Here's how the part is built. I have some questions about the finished solid (model axes, mm). A direction names the side the tool comes from. Give positions to 0.01 mm unless a question says otherwise; leave off trailing zeros. Loops run counter-clockwise (first coordinate to the right, second up) from the corner with the lowest first, then second, coordinate; pieces in that order, holes last. Notation, with made-up numbers: (-15.75, -6) -> (33.25, -6) arc R22 cw to (33.25, 11) -> close; hole circle Ø2 at (19.25, 58). An arc over 180 degrees is marked (long way). Answer in a Markdown table with one row per item. Add a question column.
Item 1: If we section it at A-A (x = -38.1): Write out the boundary of the cut face in (y, z).
Item 2: For P1, Ø3, axis at x = -21.5, z = 1.5, coming from the +Y side; P2, Ø1.9, axis at x = -72.5, z = 2.5, coming from the -Y side, each with a flat end and sliding along its axis, tell me the tip position at first contact or that it passes through.
Item 3: Which directions (+Z, -Z, +X, -X, +Y, -Y) give clear straight access to the entire face, cutting with the end or side of a thin tool? Please do faces 1 (the face through (-31.75, -3, 3)), 2 (the face through (-64, 39, 6.35)), 3 (the face through (-26, 76.2, 3)).
Item 4: If we section it at B-B (z = 1.5): Give the number of separate pieces and of enclosed holes in the cut face, then the cut area to 3 significant figures.
Item 5: We'd pull the mould along Y, two halves only. Please class faces 4 (the face through (-67, 0, 3)), 5 (the face through (-40.64, 79, 3)), 6 (the face through (-105.863, 70.44, 3.219)): released by +Y, released by -Y, zero draft, split by the parting line, or undercut.
Item 6: If I drill on line 1 (Y direction, x = -108.5, z = 2.5); line 2 (Y direction, x = -25.5, z = 2.75); line 3 (X direction, y = -0.5, z = 1.5), over which ranges is the centre line in solid material (lowest first)?
```python
from build123d import *

# Parameters (mm, degrees)
SKETCH1_W           = 127
SKETCH1_H           = 82.55
SKETCH1_R           = 10.16
SKETCH1_R_2         = 6.985
SKETCH1_W_2         = 25.4
SKETCH1_H_2         = 6.35
SKETCH1_W_3         = 31.75
BOSS_EXTRUDE1_DEPTH = 6.35
SKETCH3_R           = 2.6035
CUT_EXTRUDE1_DEPTH  = 152.604172106
SKETCH4_W           = 27.94
SKETCH4_H           = 6.35
CUT_EXTRUDE2_DEPTH  = 6.35


with BuildPart() as part:
    # Sketch1 → Boss-Extrude1 (new body)
    # profile 1 of 3: a face of its own
    with BuildSketch(Plane.XY):
        with Locations((-63.5, 41.275)):
            Rectangle(SKETCH1_W, SKETCH1_H)
        with Locations((-78.105, 41.275)):
            Circle(SKETCH1_R, mode=Mode.SUBTRACT)
        with Locations((-38.1, 41.275)):
            Circle(SKETCH1_R_2, mode=Mode.SUBTRACT)
    # profile 2 of 3: a face of its own
    with BuildSketch(Plane.XY):
        with Locations((-114.3, -3.175)):
            Rectangle(SKETCH1_W_2, SKETCH1_H_2)
    # profile 3 of 3: a face of its own
    with BuildSketch(Plane.XY):
        with Locations((-15.875, -3.175)):
            Rectangle(SKETCH1_W_3, SKETCH1_H_2)
    extrude(amount=BOSS_EXTRUDE1_DEPTH)

    # Sketch3 → Cut-Extrude1 (cut, through all)
    with BuildSketch(Plane.XY.offset(6.35)):
        with Locations((-108.2675, 71.4375)):
            Circle(SKETCH3_R)
        with Locations((-47.9425, 71.4375)):
            Circle(SKETCH3_R)
        with Locations((-108.2675, 11.1125)):
            Circle(SKETCH3_R)
        with Locations((-47.9425, 11.1125)):
            Circle(SKETCH3_R)
    extrude(amount=-CUT_EXTRUDE1_DEPTH, mode=Mode.SUBTRACT)

    # Sketch4 → Cut-Extrude2 (cut)
    with BuildSketch(Plane(origin=(0, 0, 0), x_dir=(-1, 0, 0), z_dir=(0, 0, -1))):
        with Locations((26.67, 79.375)):
            Rectangle(SKETCH4_W, SKETCH4_H)
    extrude(amount=-CUT_EXTRUDE2_DEPTH, mode=Mode.SUBTRACT)


solid = part.part
```
Recorded:
| question | item | result |
|---|---|---|
| 1 | outline | (0, 0) -> (34.29, 0) -> (34.29, 6.35) -> (0, 6.35) -> close; (48.26, 0) -> (76.2, 0) -> (76.2, 6.35) -> (48.26, 6.35) -> close |
| 2 | P1 | stops at y = 76.2 |
| 2 | P2 | stops at y = 0 |
| 3 | face 1 | +Z, -Z, -Y |
| 3 | face 2 | +Z, +X, -X, +Y, -Y |
| 3 | face 3 | +Z, -Z, +Y |
| 4 | separate pieces | 1 |
| 4 | enclosed holes | 6 |
| 4 | area | 10,100 mm^2 |
| 5 | face 4 | released by -Y |
| 5 | face 5 | zero draft |
| 5 | face 6 | undercut |
| 6 | line 1 | y = -6.35 to 8.52, 13.71 to 68.84, 74.03 to 82.55 |
| 6 | line 2 | y = -6.35 to 76.2 |
| 6 | line 3 | x = -127 to -101.6, -31.75 to 0 |
